```python
from build123d import *

# Parameters (mm, degrees)
SKETCH1_W           = 150
SKETCH1_H           = 45
BOSS_EXTRUDE1_DEPTH = 10
SKETCH2_W           = 150
SKETCH2_H           = 45
BOSS_EXTRUDE2_DEPTH = 10
SKETCH3_R           = 2.75
CUT_EXTRUDE1_DEPTH  = 30
CUT_EXTRUDE2_DEPTH  = 30
CUT_EXTRUDE3_DEPTH  = 47
SKETCH7_W           = 150
SKETCH7_H           = 125
SKETCH7_W_2         = 135
SKETCH7_H_2         = 110
BOSS_EXTRUDE3_DEPTH = 50
SKETCH8_W           = 135
SKETCH8_H           = 7.5
BOSS_EXTRUDE4_DEPTH = 110
CHAMFER2_SIZE       = 100
CHAMFER2_SIZE2      = 8.748866353


with BuildPart() as part:
    # Sketch1 → Boss-Extrude1 (new body)
    with BuildSketch(Plane.XY):
        Polygon((52.5, 45), (52.5, 170), (202.5, 170), (202.5, 45), (202.5, 0), (222.5, 0), (222.5, 190), (32.5, 190), (32.5, 45), (32.5, 0), (52.5, 0), align=None)
        with Locations((127.5, 22.5)):
            Rectangle(SKETCH1_W, SKETCH1_H)
    extrude(amount=BOSS_EXTRUDE1_DEPTH)

    # Sketch2 → Boss-Extrude2 (add)
    with BuildSketch(Plane(origin=(0, 0, 0), x_dir=(-1, 0, 0), z_dir=(0, 0, -1))):
        with Locations((-127.5, 22.5)):
            Rectangle(SKETCH2_W, SKETCH2_H)
    extrude(amount=BOSS_EXTRUDE2_DEPTH)

    # Sketch3 → Cut-Extrude1 (cut)
    with BuildSketch(Plane(origin=(0, 0, -10), x_dir=(-1, 0, 0), z_dir=(0, 0, -1))):
        with Locations((-85, 20)):
            Circle(SKETCH3_R)
    extrude(amount=-CUT_EXTRUDE1_DEPTH, mode=Mode.SUBTRACT)

    # Sketch4 → Cut-Extrude2 (cut)
    with BuildSketch(Plane.XY.offset(10)):
        with BuildLine():
            ThreePointArc((40.555456352, 181.944543648), (40.555456352, 178.055456352), (44.444543648, 178.055456352))
            Line((44.444543648, 178.055456352), (40.555456352, 181.944543648))
        make_face()
        with BuildLine():
            Line((40.555456352, 181.944543648), (44.444543648, 178.055456352))
            ThreePointArc((44.444543648, 178.055456352), (45.040668714, 178.947620561), (45.25, 180))
            ThreePointArc((45.25, 180), (43.552379439, 182.540668714), (40.555456352, 181.944543648))
        make_face()
        with BuildLine():
            ThreePointArc((130.25, 180), (129.444543648, 181.944543648), (127.5, 182.75))
            Line((127.5, 182.75), (127.5, 177.25))
            ThreePointArc((127.5, 177.25), (129.444543648, 178.055456352), (130.25, 180))
        make_face()
        with BuildLine():
            Line((127.5, 177.25), (127.5, 182.75))
            ThreePointArc((127.5, 182.75), (124.75, 180), (127.5, 177.25))
        make_face()
        with BuildLine():
            ThreePointArc((214.444543648, 181.944543648), (210.555456352, 181.944543648), (210.555456352, 178.055456352))
            Line((210.555456352, 178.055456352), (214.444543648, 181.944543648))
        make_face()
        with BuildLine():
            Line((214.444543648, 181.944543648), (210.555456352, 178.055456352))
            ThreePointArc((210.555456352, 178.055456352), (213.552379439, 177.459331286), (215.25, 180))
            ThreePointArc((215.25, 180), (215.040668714, 181.052379439), (214.444543648, 181.944543648))
        make_face()
    extrude(amount=-CUT_EXTRUDE2_DEPTH, mode=Mode.SUBTRACT)

    # Sketch5 → Cut-Extrude3 (cut)
    with BuildSketch(Plane.XY.offset(10)):
        with BuildLine():
            ThreePointArc((215.25, 22.5), (212.5, 25.25), (209.75, 22.5))
            Line((209.75, 22.5), (215.25, 22.5))
        make_face()
        with BuildLine():
            Line((215.25, 22.5), (209.75, 22.5))
            ThreePointArc((209.75, 22.5), (212.5, 19.75), (215.25, 22.5))
        make_face()
    extrude(amount=-CUT_EXTRUDE3_DEPTH, mode=Mode.SUBTRACT)

    # Sketch7 → Boss-Extrude3 (add)
    with BuildSketch(Plane.XY.offset(10)):
        with Locations((127.5, 107.5)):
            Rectangle(SKETCH7_W, SKETCH7_H)
        with Locations((127.5, 107.5)):
            Rectangle(SKETCH7_W_2, SKETCH7_H_2, mode=Mode.SUBTRACT)
    extrude(amount=-BOSS_EXTRUDE3_DEPTH)

    # Sketch8 → Boss-Extrude4 (add)
    with BuildSketch(Plane.XZ.offset(-162.5)):
        with Locations((127.5, -36.25)):
            Rectangle(SKETCH8_W, SKETCH8_H)
    extrude(amount=BOSS_EXTRUDE4_DEPTH)

    # Chamfer2
    chamfer2_edges = [part.edges().sort_by_distance(p)[0] for p in [
        (195, 107.5, -32.5),
        (127.5, 52.5, -32.5),
    ]]
    chamfer2_side = [part.faces().sort_by_distance(p)[0] for p in [
        (127.5, 107.5, -32.5),
    ]]
    chamfer(chamfer2_edges, length=CHAMFER2_SIZE, length2=CHAMFER2_SIZE2, reference=chamfer2_side[0])


solid = part.part
```
The listing builds one solid part. Answer for the finished solid, in the listing's coordinates (mm). A direction names the side the tool comes from. Give positions to 0.01 mm unless a question says otherwise; leave off trailing zeros. Order: outer loops, then holes, each group sorted by start corner. A loop starts at its lowest first (then second) coordinate and runs counter-clockwise, first axis right, second up. Notation, with made-up numbers: (35.25, 66.25) - (85.25, 66.25) arc R18 ccw to (85.25, 89.25) - close; hole circle Ø8 at (54.5, 10.5). An arc over 180 degrees is marked (long way). Answer in a Markdown table with one row per item. Add a question column.
Q1. For a pull along Y with two mould halves and no side action, classify faces 1 (the flat face through (126, 45, -25)), 2 (the flat face through (126, 170, -20)), 3 (the flat face through (126, 108, -40)), 4 (the flat face through (127, 162.5, -11)) as released by +Y, released by -Y, zero draft, split by the parting line, or undercut.
Q2. The part is cut by section D-D (x = 116.5). Determine the outline of the cut face in (y, z).
Q3. Find the intervals of material crossed by line 1 along Y through (x, z) = (85, 2); line 2 along Y through (x, z) = (85, -1); line 3 along Y through (x, z) = (147, 0.5), in increasing order. Write a range as [from, to].
Q4. Which of the six approach directions +Z, -Z, +X, -X, +Y, -Y give full straight-line access (tool end or side, diameter ignored) to faces 5 (the flat face through (202.5, 103, -20)), 6 (the flat face through (156.811, 120.492, -27.092)), 7 (the flat face through (52.5, 103, -20))?
Q5. Given P1, Ø17, axis at y = 100.5, z = -15, coming from the -X side; P2, Ø1, axis at y = 162, z = -13.5, coming from the +X side; P3, Ø5, axis at x = 81, y = 155, coming from the +Z side; P4, Ø6, axis at x = 152.5, z = -6.5, coming from the -Y side, each flat-ended and moving along its own axis, determine where each tip first touches the part or whether it passes through.
Q6. The part is cut by section A-A (x = 85). Determine the outline of the cut face in (y, z), then the cut area to 3 significant figures.
Q7. The part is cut by section C-C (y = 123). Determine the outline of the cut face in (x, z).
Q8. The part is cut by section B-B (z = -16.5). Determine the outline of the cut face in (x, y).
Determined:
| question | item | result |
|---|---|---|
| 1 | face 1 | released by -Y |
| 1 | face 2 | released by +Y |
| 1 | face 3 | zero draft |
| 1 | face 4 | undercut |
| 2 | outline | (0, -10) - (45, -10) - (45, -40) - (170, -40) - (170, 0) - (190, 0) - (190, 10) - (162.5, 10) - (162.5, -30.62) - (131, -30.62) - (52.5, -23.75) - (52.5, 10) - (0, 10) - close |
| 3 | line 1 | y = [0, 17.25], [22.75, 52.5], [162.5, 190] |
| 3 | line 2 | y = [0, 17.25], [22.75, 52.5], [162.5, 170] |
| 3 | line 3 | y = [0, 52.5], [162.5, 190] |
| 4 | face 5 | -Z, +X, +Y, -Y |
| 4 | face 6 | +Z |
| 4 | face 7 | -Z, -X, +Y, -Y |
| 5 | P1 | stops at x = 52.5 |
| 5 | P2 | stops at x = 202.5 |
| 5 | P3 | stops at z = -32.5 |
| 5 | P4 | stops at y = 0 |
| 6 | outline | (0, -10) - (17.25, -10) - (17.25, 10) - (0, 10) - close; (22.75, -10) - (45, -10) - (45, -40) - (170, -40) - (170, 0) - (190, 0) - (190, 10) - (162.5, 10) - (162.5, -32.5) - (152.5, -32.5) - (52.5, -23.75) - (52.5, 10) - (22.75, 10) - close |
| 6 | area | 3,000 mm² |
| 7 | outline | (32.5, 0) - (52.5, 0) - (52.5, -40) - (202.5, -40) - (202.5, 0) - (222.5, 0) - (222.5, 10) - (195, 10) - (195, -23.75) - (124.5, -29.92) - (60, -29.92) - (60, 10) - (32.5, 10) - close |
| 8 | outline | (52.5, 45) - (202.5, 45) - (202.5, 170) - (52.5, 170) - close; hole (60, 52.5) - (195, 52.5) - (195, 162.5) - (60, 162.5) - close |
